Autodesk Fusion 360 part; units mm, degrees
sketch "Sketch1" plane through (0, 0, 0) normal (0, 0, 1) x (1, 0, 0)
  line L0 (-6.05, -8.5) -> (-6.05, 0)
  line L1 (-6.05, 0) -> (6.05, 0)
  line L2 (6.05, 0) -> (6.05, -8.5)
  line L3 (6.05, -8.5) -> (10.05, -8.5)
  line L4 (10.05, -8.5) -> (10.05, -18.5)
  line L5 (-6.05, -8.5) -> (-10.05, -8.5)
  line L6 (-10.05, -8.5) -> (-10.05, -18.5)
  line L7 (10.05, -18.5) -> (15.05, -18.5)
  line L8 (15.05, -18.5) -> (15.05, 6.5)
  line L9 (15.05, 6.5) -> (-15.05, 6.5)
  line L10 (-15.05, 6.5) -> (-15.05, -18.5)
  line L11 (-15.05, -18.5) -> (-10.05, -18.5)
  arc A0 (-10.05, 6.5) -> (-15.05, 1.5) centre (-10.05, 1.5) ccw
  arc A1 (15.05, 1.5) -> (10.05, 6.5) centre (10.05, 1.5) ccw
  line L12 (-10.05, -18.5) -> (10.05, -18.5) construction
  point P0 (0, -18.5)
  dimension "d1" = 12.1
  dimension "d2" = 8.5
  dimension "d3" = 20.1
  dimension "d4" = 10
  dimension "d5" = 5
  dimension "d6" = 25
  dimension "d7" = 5
  dimension "d8" = 5
extrude "Extrude1" add sketch "Sketch1" along normal blind 8 contours L0 L1 L2 L3 L4 L5 L6 L7 L8 L9 L10 L11 A0 A1
fillet "Fillet1" radius 1 10 edges at (6.05, 0, 4) (-6.05, 0, 4) (-6.05, -8.5, 4) (-10.05, -8.5, 4) (-10.05, -18.5, 4) (-15.05, -18.5, 4) (6.05, -8.5, 4) (10.05, -8.5, 4) (10.05, -18.5, 4) (15.05, -18.5, 4)
chamfer "Chamfer1" distance 0.4 angle 45 48 edges at (12.55, -18.5, 0) (14.7571, -18.2071, 0) (15.05, -8, 0) (13.5855, 5.0355, 0) (0, 6.5, 0) (-13.5855, 5.0355, 0) (-15.05, -8, 0) (-14.7571, -18.2071, 0) (-12.55, -18.5, 0) (-10.3429, -18.2071, 0) (-10.05, -13.5, 0) (-9.7571, -8.7929, 0) (-8.05, -8.5, 0) (-6.3429, -8.2071, 0) (-6.05, -4.25, 0) (-5.7571, -0.2929, 0) (0, 0, 0) (5.7571, -0.2929, 0) (6.05, -4.25, 0) (6.3429, -8.2071, 0) (8.05, -8.5, 0) (9.7571, -8.7929, 0) (10.05, -13.5, 0) (10.3429, -18.2071, 0) (12.55, -18.5, 8) (14.7571, -18.2071, 8) (15.05, -8, 8) (13.5855, 5.0355, 8) (0, 6.5, 8) (-13.5855, 5.0355, 8) (-15.05, -8, 8) (-14.7571, -18.2071, 8) (-12.55, -18.5, 8) (-10.3429, -18.2071, 8) (-10.05, -13.5, 8) (-9.7571, -8.7929, 8) (-8.05, -8.5, 8) (-6.3429, -8.2071, 8) (-6.05, -4.25, 8) (-5.7571, -0.2929, 8) (0, 0, 8) (5.7571, -0.2929, 8) (6.05, -4.25, 8) (6.3429, -8.2071, 8) (8.05, -8.5, 8) (9.7571, -8.7929, 8) (10.05, -13.5, 8) (10.3429, -18.2071, 8)
Model file for the job. Use its own axes, mm. A direction names the side the tool comes from. Give positions to 0.01 mm unless a question says otherwise; leave off trailing zeros. Loops run counter-clockwise (first coordinate to the right, second up) from the corner with the lowest first, then second, coordinate; pieces in that order, holes last.
Item 1: Slice it at D-D (y = -11). Write the cut outline in (x, z).
Check values:
outline: (-15.05, 0.4) - (-14.65, 0) - (-10.45, 0) - (-10.05, 0.4) - (-10.05, 7.6) - (-10.45, 8) - (-14.65, 8) - (-15.05, 7.6) - close; (10.05, 0.4) - (10.45, 0) - (14.65, 0) - (15.05, 0.4) - (15.05, 7.6) - (14.65, 8) - (10.45, 8) - (10.05, 7.6) - close
Item 2: Mould opens along X. For faces 1 (the face through (6.508, -8.03, 0.158)), 2 (the face through (-13.62, 5, 3.95)), 3 (the face through (0, 6.5, 4)) say: +X half, -X half, draft (parallel to the pull), parting line (faces both ways), or undercut.
Check values:
face 1: undercut
face 2: -X half
face 3: draft
Item 3: Drill centre lines: line 1 along X through (y, z) = (-6.5, 3.75); line 2 along X through (y, z) = (-12.5, 4.5); line 3 along Y through (x, z) = (-1, 0.75). Where is each one in solid material? Low to high.
Check values:
line 1: x = -15.05 to -6.05, 6.05 to 15.05
line 2: x = -15.05 to -10.05, 10.05 to 15.05
line 3: y = 0 to 6.5
Item 4: Slice it at C-C (z = 6.5). Write the cut outline in (x, y).
Check values:
outline: (-15.05, -17.5) arc R1 ccw to (-14.05, -18.5) - (-11.05, -18.5) arc R1 ccw to (-10.05, -17.5) - (-10.05, -9.5) arc R1 cw to (-9.05, -8.5) - (-7.05, -8.5) arc R1 ccw to (-6.05, -7.5) - (-6.05, -1) arc R1 cw to (-5.05, 0) - (5.05, 0) arc R1 cw to (6.05, -1) - (6.05, -7.5) arc R1 ccw to (7.05, -8.5) - (9.05, -8.5) arc R1 cw to (10.05, -9.5) - (10.05, -17.5) arc R1 ccw to (11.05, -18.5) - (14.05, -18.5) arc R1 ccw to (15.05, -17.5) - (15.05, 1.5) arc R5 ccw to (10.05, 6.5) - (-10.05, 6.5) arc R5 ccw to (-15.05, 1.5) - close
Item 5: Which spindle directions (+Z, -Z, +X, -X, +Y, -Y) get a long thin tool onto all of the face, cutting with end or side? Do faces 4 (the face through (13.346, 4.87, 7.886)), 5 (the face through (-10.52, -18.042, 0.158)), 6 (the face through (-6.05, -4, 4)), 7 (the face through (-13.42, 4.796, 7.886)), 8 (the face through (6.52, -8.042, 7.842)). Say none if no direction does.
Check values:
face 4: +Z, +X, +Y
face 5: -Z, -Y
face 6: +Z, -Z, -Y
face 7: +Z, -X, +Y
face 8: +Z, -Y
Item 6: Slice it at B-B (x = -1.5). Write the cut outline in (y, z), plus the area to 3 significant figures.
Check values:
outline: (0, 0.4) - (0.4, 0) - (6.1, 0) - (6.5, 0.4) - (6.5, 7.6) - (6.1, 8) - (0.4, 8) - (0, 7.6) - close
area: 51.7 mm2
Item 7: Drop flat-ended pins along their axis: P1, Ø1, axis at x = 7.5, z = 5, coming from the -Y side; P2, Ø3, axis at x = 3, z = 2.5, coming from the -Y side. Give the stop position or say it passes through.
Check values:
P1: stops at y = -8.5
P2: stops at y = 0
Item 8: Slice it at A-A (y = -4.75). Write the cut outline in (x, z), plus the area to 3 significant figures.
Check values:
outline: (-15.05, 0.4) - (-14.65, 0) - (-6.45, 0) - (-6.05, 0.4) - (-6.05, 7.6) - (-6.45, 8) - (-14.65, 8) - (-15.05, 7.6) - close; (6.05, 0.4) - (6.45, 0) - (14.65, 0) - (15.05, 0.4) - (15.05, 7.6) - (14.65, 8) - (6.45, 8) - (6.05, 7.6) - close
area: 143 mm2
